Job drawing, mm, ordinate dimensions from the low corner. One solid piece. A direction names the side the tool comes from. Round coordinates to 2 decimals unless told otherwise and drop trailing zeros. Loops run counter-clockwise (first coordinate to the right, second up) from the corner with the lowest first, then second, coordinate; pieces in that order, holes last.
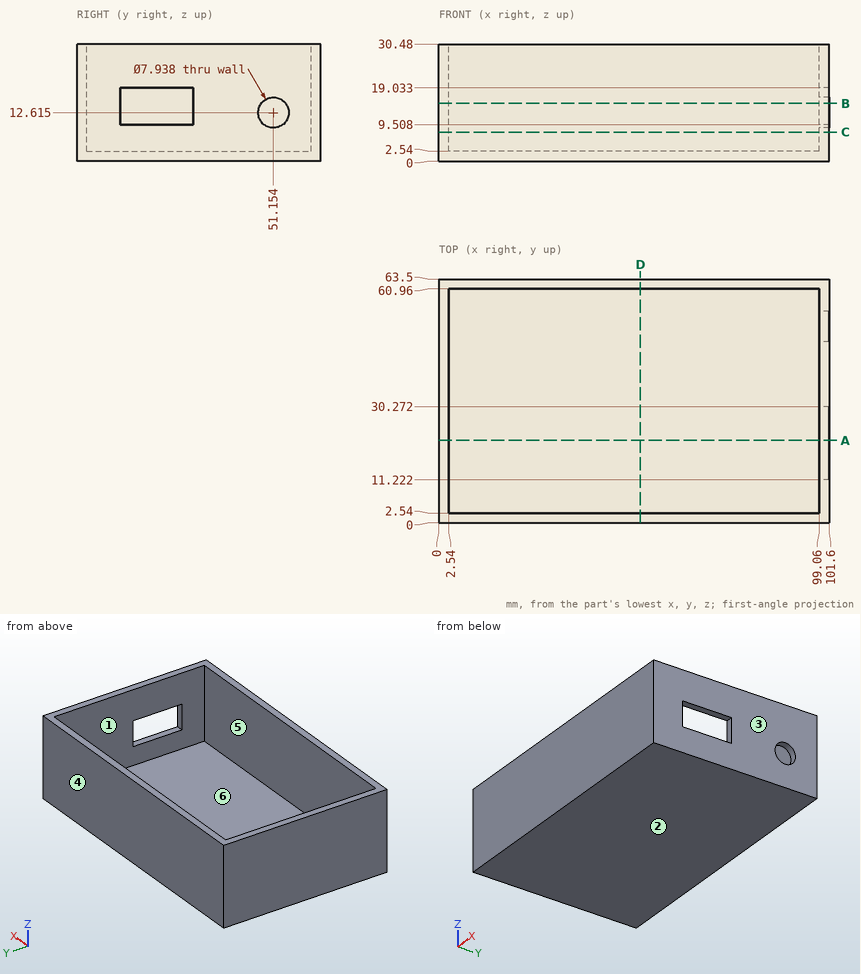
Item 1: Flat gauge pin, fed straight in: P1, Ø4, axis at x = 90, y = 22.5, coming from the +Z side. Where does the tip first touch, or does it go through?
Answers follow:
P1: stops at z = 2.54
Item 2: Two-plate mould, pull along Y, no slides. Class the marked faces 3, 4, 5 and 6: released by +Y, released by -Y, zero draft, split by the parting line, or undercut.
Answers follow:
face 3: zero draft
face 4: released by +Y
face 5: undercut
face 6: undercut
Item 3: Cut at A-A, the plane y = 21.5. Give the cut face in (x, z).
Answers follow:
outline: (0, 0) - (101.6, 0) - (101.6, 9.51) - (99.06, 9.51) - (99.06, 2.54) - (2.54, 2.54) - (2.54, 30.48) - (0, 30.48) - close; (99.06, 19.03) - (101.6, 19.03) - (101.6, 30.48) - (99.06, 30.48) - close
Item 4: Probe line 1 (X direction, y = 38, z = 26); line 2 (Y direction, x = 8.5, z = 20.5); line 3 (Z direction, x = 24.5, y = 29.5). List the from-to ranges inside material, lowest first.
Answers follow:
line 1: x = 0 to 2.54, 99.06 to 101.6
line 2: y = 0 to 2.54, 60.96 to 63.5
line 3: z = 0 to 2.54
Item 5: Cut at C-C, the plane z = 7.5. Give the cut face in (x, y).
Answers follow:
outline: (0, 0) - (101.6, 0) - (101.6, 63.5) - (0, 63.5) - close; hole (2.54, 2.54) - (99.06, 2.54) - (99.06, 60.96) - (2.54, 60.96) - close
Item 6: Cut at D-D, the plane x = 52.5. Give the cut face in (y, z), plus the area to 3 significant figures.
Answers follow:
outline: (0, 0) - (63.5, 0) - (63.5, 30.48) - (60.96, 30.48) - (60.96, 2.54) - (2.54, 2.54) - (2.54, 30.48) - (0, 30.48) - close
area: 303 mm2
Item 7: 3-axis set-ups, long thin cutter, end or side, ignore diameter. For the marked faces 1 and 2: which of +Z, -Z, +X, -X, +Y, -Y reach the whole face in a straight line?
Answers follow:
face 1: +Z
face 2: -Z, +X, -X, +Y, -Y
Item 8: Cut at B-B, the plane z = 15. Give the cut face in (x, y) (1 decimal).
Answers follow:
outline: (0, 0) - (101.6, 0) - (101.6, 11.2) - (99.1, 11.2) - (99.1, 2.5) - (2.5, 2.5) - (2.5, 61) - (99.1, 61) - (99.1, 54.3) - (101.6, 54.3) - (101.6, 63.5) - (0, 63.5) - close; (99.1, 30.3) - (101.6, 30.3) - (101.6, 48) - (99.1, 48) - close
